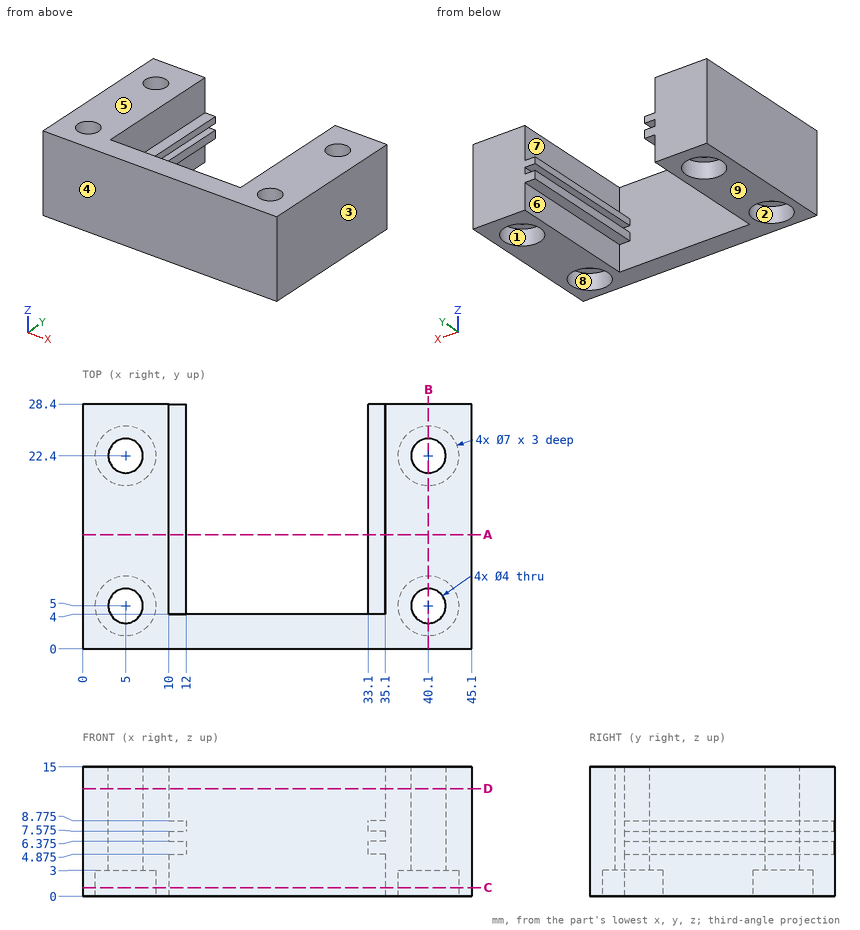
Verification items for this drawing (mm, ordinates from the low corner). A direction names the side the tool comes from. Round coordinates to 2 decimals unless told otherwise and drop trailing zeros. Order: outer loops, then holes, each group sorted by start corner. A loop starts at its lowest first (then second) coordinate and runs counter-clockwise, first axis right, second up. Notation, with made-up numbers: (55, 8.25) - (85, 8.25) arc R22 ccw to (85, 29.25) - close; hole circle Ø6 at (-7, 17.5). An arc over 180 degrees is marked (long way). Use CSV: the item, a comma, the result in double quotes.
(1) Thickness scan on probe 1 along Y at (x, z) = (40.1, 11.25); probe 2 along Y at (x, z) = (40.1, 1.9); probe 3 along X at (y, z) = (12, 1.5). Record the ranges inside material, lowest first. Write a range as from..to.
Entries:
probe 1,"0..3, 7..20.4, 24.4..28.4"
probe 2,"0..1.5, 8.5..18.9, 25.9..28.4"
probe 3,"0..10, 35.1..45.1"
(2) Section check D-D on z = 12.5. Record the boundary of the cut face in (x, y).
Entries:
outline,"(0, 0) - (45.1, 0) - (45.1, 28.4) - (35.1, 28.4) - (35.1, 4) - (10, 4) - (10, 28.4) - (0, 28.4) - close; hole circle Ø4 at (5, 5); hole circle Ø4 at (5, 22.4); hole circle Ø4 at (40.1, 5); hole circle Ø4 at (40.1, 22.4)"
(3) Gauge pin test, flat ends, axial feed: pin 1 Ø1.5 at (x, z) = (29, 7.5) entering from +Y; pin 2 Ø1.6 at (x, y) = (11.5, 16) entering from +Z (3 decimals); pin 3 Ø6.5 at (x, y) = (40.1, 5) entering from -Z. Record the tip position at first contact, or that the pin passes through.
Entries:
pin 1,"y = 4"
pin 2,"z = 8.775"
pin 3,"z = 3"
(4) Section check C-C on z = 1. Record the boundary of the cut face in (x, y).
Entries:
outline,"(0, 0) - (45.1, 0) - (45.1, 28.4) - (35.1, 28.4) - (35.1, 4) - (10, 4) - (10, 28.4) - (0, 28.4) - close; hole circle Ø7 at (5, 5); hole circle Ø7 at (5, 22.4); hole circle Ø7 at (40.1, 5); hole circle Ø7 at (40.1, 22.4)"
(5) Section check B-B on x = 40.1. Record the boundary of the cut face in (y, z).
Entries:
outline,"(0, 0) - (1.5, 0) - (1.5, 3) - (3, 3) - (3, 15) - (0, 15) - close; (7, 3) - (8.5, 3) - (8.5, 0) - (18.9, 0) - (18.9, 3) - (20.4, 3) - (20.4, 15) - (7, 15) - close; (24.4, 3) - (25.9, 3) - (25.9, 0) - (28.4, 0) - (28.4, 15) - (24.4, 15) - close"
(6) Section check A-A on y = 13.25. Record the boundary of the cut face in (x, z) (3 decimals), and give its area (3 significant figures).
Entries:
outline,"(0, 0) - (10, 0) - (10, 4.875) - (12, 4.875) - (12, 6.375) - (10, 6.375) - (10, 7.575) - (12, 7.575) - (12, 8.775) - (10, 8.775) - (10, 15) - (0, 15) - close; (33.1, 4.875) - (35.1, 4.875) - (35.1, 0) - (45.1, 0) - (45.1, 15) - (35.1, 15) - (35.1, 8.775) - (33.1, 8.775) - (33.1, 7.575) - (35.1, 7.575) - (35.1, 6.375) - (33.1, 6.375) - close"
area,"311 mm^2"
(7) Access from +Z, -Z, +X, -X, +Y, -Y to the whole of each face (thin tool, end or side, straight path). Record for the marked faces 5, 6, 7, 8 and 9.
Entries:
face 5,"+Z, +X, -X, +Y, -Y"
face 6,"-Z, +Y"
face 7,"+Z, +Y"
face 8,"-Z"
face 9,"-Z, +X, -X, +Y, -Y"
(8) Mould release check, pull along Y, two halves, no side actions. Record for the marked faces 1, 2, 3 and 4: released by +Y, released by -Y, zero draft, split by the parting line, or undercut.
Entries:
face 1,"undercut"
face 2,"undercut"
face 3,"zero draft"
face 4,"released by -Y"
